Input: dimensioned drawing with shaded views. Units: mm. Origin: part minimum x, y, z. Round coordinates to 2 decimals unless told otherwise and drop trailing zeros. Loops run counter-clockwise (first coordinate to the right, second up) from the corner with the lowest first, then second, coordinate; pieces in that order, holes last.
1) Ray query, line 1 along Y through (x, z) = (35, 34); line 2 along Y through (x, z) = (37.5, 49.5) (1 decimal); line 3 along Z through (x, y) = (14, 16.5). Return the intervals inside material, ascending.
2) First-contact query: pin 1 (8 mm diameter, centred on x = 22.5, y = 11, fed in from -Z); pin 2 (8 mm diameter, centred on x = 32, y = 30, fed in from +Z); pin 3 (4 mm diameter, centred on x = 36.5, y = 21, fed in from -Z). Flat tips, straight axial feed; report the tip coordinate or a pass-through.
3) Section D-D, the plane x = 4. Return loops of the section in (y, z).
4) Draft query along Z for the marked faces 1, 2 and 3. Return one class per face: pulls with the +Z half, pulls with the -Z half, needs draft (parallel to the pull), parting line crosses it, or undercut.
5) Section B-B, the plane z = 34. Return loops of the section in (x, y).
6) Section A-A, the plane y = 34. Return loops of the section in (x, z).
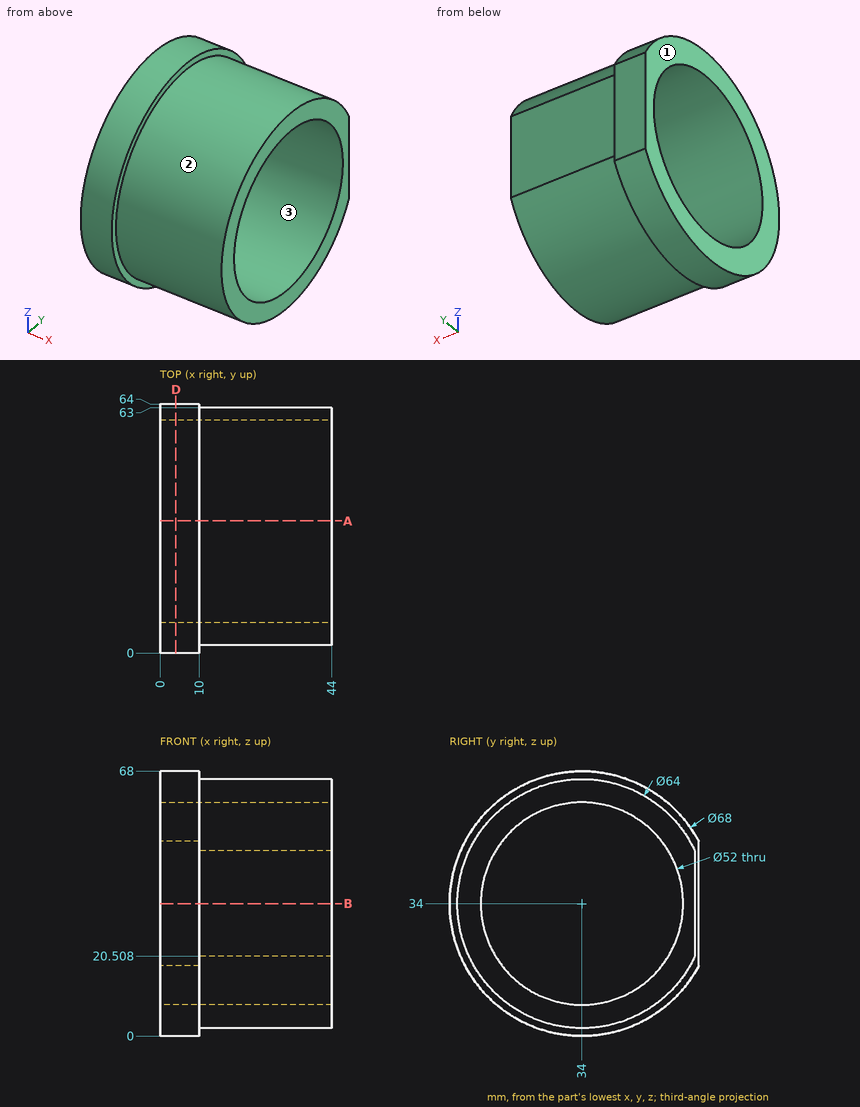
Final values:
1. line 1: y = 2 to 8, 60 to 63
1. line 2: y = 6 to 13.1, 54.9 to 62
1. line 3: z = 7.21 to 14.77, 53.23 to 60.79
2. pin 1: stops at z = 8.25
2. pin 2: stops at z = 66
2. pin 3: stops at z = 3.95
3. outline: (64, 18) - (64, 50) arc R34 ccw (long way) to start; hole circle Ø52 at (34, 34)
4. face 1: needs draft
4. face 2: parting line crosses it
4. face 3: undercut
5. outline: (0, 0) - (10, 0) - (10, 2) - (44, 2) - (44, 8) - (0, 8) - close; (0, 60) - (44, 60) - (44, 63) - (10, 63) - (10, 64) - (0, 64) - close
6. outline: (0, 0) - (10, 0) - (10, 2) - (44, 2) - (44, 8) - (0, 8) - close; (0, 60) - (44, 60) - (44, 66) - (10, 66) - (10, 68) - (0, 68) - close
